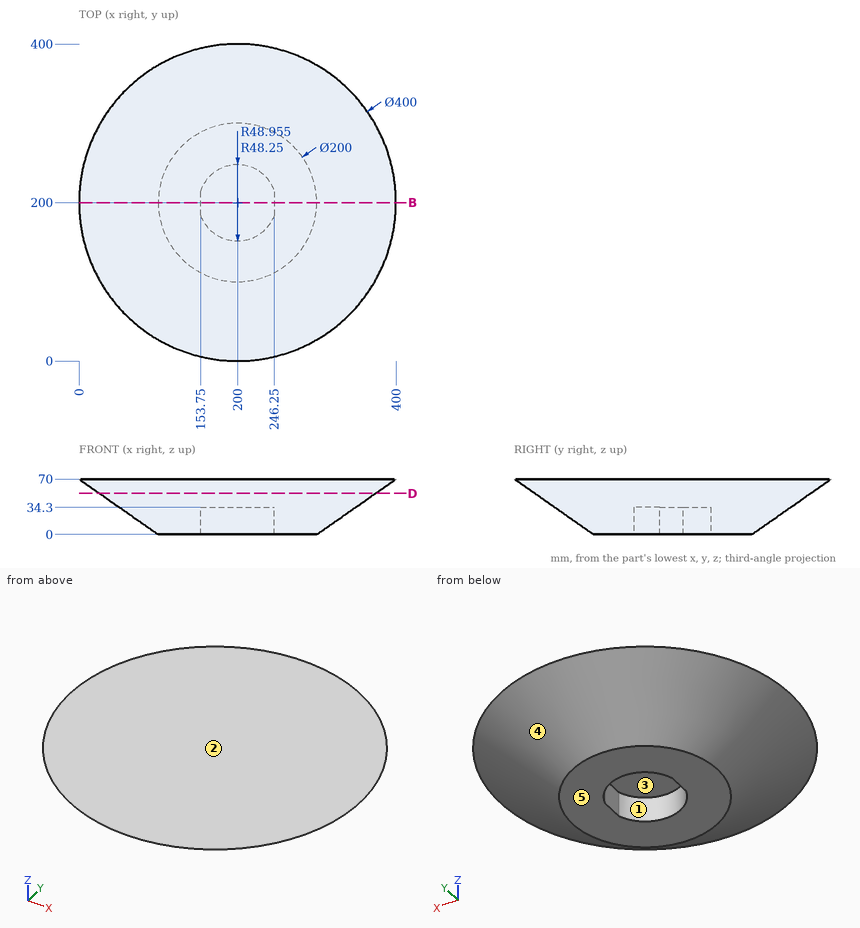
The figure shows three views and two pictorial views of one solid part (mm, origin at its lowest corner). Answer the questions. A direction names the side the tool comes from. Give positions to 0.01 mm unless a question says otherwise; leave off trailing zeros. Write each loop counter-clockwise with the first axis right and the second up, starting at its lowest first coordinate (ties: lowest second). Pieces come first, ordered by that corner, then holes. Notation, with made-up numbers: (10.25, 61.5) -> (49.25, 61.5) arc R24 cw to (49.25, 86.5) -> close; hole circle Ø10 at (-27.75, -7). An arc over 180 degrees is marked (long way). Answer as a JSON object with one key per item and string values.
1) For a pull along X with two mould halves and no side action, classify the marked faces 3, 4 and 5 as pulls with the +X half, pulls with the -X half, needs draft (parallel to the pull), parting line crosses it, or undercut.
Findings below:
{"face 3": "undercut", "face 4": "parting line crosses it", "face 5": "needs draft"}
2) Section B-B on y = 200 is taken. Write down the section's boundary in (x, z), then the cut area to 3 significant figures.
Findings below:
{"outline": "(0, 70) -> (100, 0) -> (153.75, 0) -> (153.75, 34.3) -> (246.25, 34.3) -> (246.25, 0) -> (300, 0) -> (400, 70) -> close", "area": "17,800 mm^2"}
3) Section D-D on z = 52 is taken. Write down the section's boundary in (x, y).
Findings below:
{"outline": "circle Ø348.57 at (200, 200)"}
4) A tool of negligible diameter and unlimited length cuts with its end or side. For the marked faces 1 and 2, from which of +Z, -Z, +X, -X, +Y, -Y can it reach the whole face along a straight path? Write none if from no direction.
Findings below:
{"face 1": "-Z", "face 2": "+Z, +X, -X, +Y, -Y"}
5) Flat-ended cylindrical pins translate along their axes: pin 1 Ø3 at (x, z) = (158.5, 35.5) entering from -Y (1 decimal); pin 2 Ø2 at (y, z) = (127, 28) entering from -X; pin 3 Ø6 at (y, z) = (148.5, 39) entering from +X. Find the tip coordinate at first contact, or state that the pin passes through.
Findings below:
{"pin 1": "stops at y = 52.8", "pin 2": "stops at x = 78.76", "pin 3": "stops at x = 351.6"}
6) Straight lines are drawn through the part: probe 1 along X at (y, z) = (167, 6) (1 decimal); probe 2 along Z at (x, y) = (207.5, 184); probe 3 along X at (y, z) = (241.5, 11) (1 decimal). For each, find the intervals that lie inside material, in ascending order. Write a range as from..to.
Findings below:
{"probe 1": "x = 96.6..163.8, 236.2..303.4", "probe 2": "z = 34.3..70", "probe 3": "x = 92..175.4, 224.6..308"}
